Here's how the part is built. I have some questions about the finished solid (model axes, mm). A direction names the side the tool comes from. Round coordinates to 2 decimals unless told otherwise and drop trailing zeros. Write each loop counter-clockwise with the first axis right and the second up, starting at its lowest first coordinate (ties: lowest second). Pieces come first, ordered by that corner, then holes. Notation, with made-up numbers: (-27, 26) -> (17, 26) arc R25 ccw to (17, 41) -> close; hole circle Ø7 at (37.5, 64.5). An arc over 180 degrees is marked (long way). Put each result on its own line as item: value. Start each with the question number.
1) I want a section at D-D, the plane x = -1. List the corners of the cut face in (y, z) for me, then the cut area to 3 significant figures.
2) If I drill on line 1 along X through (y, z) = (3.8, 0); line 2 along Z through (x, y) = (50, 2.7); line 3 along Z through (x, y) = (9, 1.05), over which ranges is the centre line in solid material (lowest first)? Write a range as [from, to].
3) I want a section at C-C, the plane x = 9. List the corners of the cut face in (y, z) for me.
4) Will these pins go through, and if not, where does the flat tip stop? P1, Ø5, axis at x = 27.5, z = 0, coming from the -Y side; P2, Ø1.5, axis at y = 4, z = 1, coming from the -X side; P3, Ø2.5, axis at x = 50, z = 0, coming from the +Y side.
5) Which directions (+Z, -Z, +X, -X, +Y, -Y) give clear straight access to the entire face, cutting with the end or side of a thin tool? Please do faces 1 (the flat face through (44, 3, 0)), 2 (the flat face through (25, 0, 0)).
6) I want a section at B-B, the plane y = 0.65. List the corners of the cut face in (x, z) for me, then the cut area to 3 significant figures.
7) We'd pull the mould along Z, two halves only. Please class faces 3 (the cylindrical face through (48.5, 2.46, -0.07)), 4 (the flat face through (25, 5, 0)), 5 (the cylindrical face through (-4.61, 2.46, 0.1)), 6 (the flat face through (25, 2, 4.611)): released by +Z, released by -Z, zero draft, split by the parting line, or undercut.
8) I want a section at A-A, the plane z = 0. List the corners of the cut face in (x, y) for me.
from build123d import *

# Parameters (mm, degrees)
SKETCH1_R           = 1.5
BOSS_EXTRUDE1_DEPTH = 5
CUT_EXTRUDE2_DEPTH  = 17
FILLET1_R           = 1


with BuildPart() as part:
    # Sketch1 → Boss-Extrude1 (new body)
    with BuildSketch(Plane(origin=(0, 0, 0), x_dir=(1, 0, 0), z_dir=(0, 1, 0))):
        with BuildLine():
            Line((0, 4.610590887), (50, 4.610590887))
            ThreePointArc((50, 4.610590887), (54.610590887, 0), (50, -4.610590887))
            Line((50, -4.610590887), (0, -4.610590887))
            ThreePointArc((0, -4.610590887), (-4.610590887, 0), (0, 4.610590887))
        make_face()
        Circle(SKETCH1_R, mode=Mode.SUBTRACT)
        with Locations((50, 0)):
            Circle(SKETCH1_R, mode=Mode.SUBTRACT)
    extrude(amount=BOSS_EXTRUDE1_DEPTH)

    # Sketch3 → Cut-Extrude2 (cut)
    with BuildSketch(Plane(origin=(0, 5, 0), x_dir=(1, 0, 0), z_dir=(0, 1, 0))):
        Polygon((6, 2), (6, -2), (13, 0), align=None)
        Polygon((44, 2), (44, -2), (37, 0), align=None)
    extrude(amount=-CUT_EXTRUDE2_DEPTH, mode=Mode.SUBTRACT)

    # Fillet1
    fillet1_edges = [part.edges().sort_by_distance(p)[0] for p in [
        (6, 2.5, -2),
        (13, 2.5, 0),
        (6, 2.5, 2),
        (37, 2.5, 0),
        (44, 2.5, -2),
        (44, 2.5, 2),
    ]]
    fillet(fillet1_edges, radius=FILLET1_R)


solid = part.part
Findings:
1. outline: (0, -4.5) -> (5, -4.5) -> (5, -1.12) -> (0, -1.12) -> close; (0, 1.12) -> (5, 1.12) -> (5, 4.5) -> (0, 4.5) -> close
1. area: 33.8 mm2
2. line 1: x = [-4.61, -1.5], [1.5, 6], [10.36, 39.64], [44, 48.5], [51.5, 54.61]
2. line 2: z = [-4.61, -1.5], [1.5, 4.61]
2. line 3: z = [-4.61, -1.14], [1.14, 4.61]
3. outline: (0, -4.61) -> (5, -4.61) -> (5, -1.14) -> (0, -1.14) -> close; (0, 1.14) -> (5, 1.14) -> (5, 4.61) -> (0, 4.61) -> close
4. P1: stops at y = 0
4. P2: stops at x = -4.6
4. P3: passes through
5. face 1: +Y, -Y
5. face 2: +Z, -Z, +X, -X, -Y
6. outline: (0, -4.61) -> (50, -4.61) arc R4.61 ccw to (50, 4.61) -> (0, 4.61) arc R4.61 ccw to start; hole circle Ø3 at (0, 0); hole (6, -0.67) arc R1 ccw to (7.27, -1.64) -> (9.63, -0.96) arc R1 ccw to (9.63, 0.96) -> (7.27, 1.64) arc R1 ccw to (6, 0.67) -> close; hole (40.37, -0.96) -> (42.73, -1.64) arc R1 ccw to (44, -0.67) -> (44, 0.67) arc R1 ccw to (42.73, 1.64) -> (40.37, 0.96) arc R1 ccw to start; hole circle Ø3 at (50, 0)
6. area: 492 mm2
7. face 3: undercut
7. face 4: zero draft
7. face 5: split by the parting line
7. face 6: released by +Z
8. outline: (-4.61, 0) -> (-1.5, 0) -> (-1.5, 5) -> (-4.61, 5) -> close; (1.5, 0) -> (6, 0) -> (6, 5) -> (1.5, 5) -> close; (10.36, 0) -> (39.64, 0) -> (39.64, 5) -> (10.36, 5) -> close; (44, 0) -> (48.5, 0) -> (48.5, 5) -> (44, 5) -> close; (51.5, 0) -> (54.61, 0) -> (54.61, 5) -> (51.5, 5) -> close
